from build123d import *

# Parameters (mm, degrees)
SKETCH1_R           = 35.00000000000001
BOSS_EXTRUDE1_DEPTH = 12
SKETCH2_R           = 38
CUT_EXTRUDE1_DEPTH  = 7.825
SKETCH3_R           = 40.5
CUT_EXTRUDE2_DEPTH  = 5
BOSS_EXTRUDE3_START = -3
SKETCH4_R           = 50.000000000000014
SKETCH4_R_2         = 40.5
BOSS_EXTRUDE3_DEPTH = 3
FILLET1_R           = 10
SKETCH5_R           = 2.5000000000000018
CUT_EXTRUDE3_DEPTH  = 72.72168430816446
CUT_EXTRUDE4_REACH  = 73.722
SKETCH9_R           = 3.999999999999999
CHAMFER2_SIZE       = 2.5
CHAMFER2_SIZE2      = 5.361267301273932
SKETCH10_R          = 2.499999999999999
SKETCH10_R_2        = 2.5000000000000004
SKETCH10_R_3        = 2.5000000000000018
SKETCH10_R_4        = 2.499999999999998
CUT_EXTRUDE5_DEPTH  = 7


with BuildPart() as part:
    # Sketch1 → Boss-Extrude1 (new body)
    with BuildSketch(Plane(origin=(0, 0, 0), x_dir=(0, 0, -1), z_dir=(1, 0, 0))):
        with BuildLine():
            Line((-0.9297857327654514, 49.99135423741935), (0.9297857327657116, 49.99135423741935))
            ThreePointArc((0.9297857327657116, 49.99135423741935), (50, 4.17e-15), (0.9297857327657116, -49.99135423741935))
            Line((0.9297857327657116, -49.99135423741935), (-0.9297857327654514, -49.99135423741935))
            ThreePointArc((-0.9297857327654514, -49.99135423741935), (-50.00000000000001, 1.029e-14), (-0.9297857327654514, 49.99135423741935))
        make_face()
        Circle(SKETCH1_R, mode=Mode.SUBTRACT)
    extrude(amount=BOSS_EXTRUDE1_DEPTH)

    # Sketch2 → Cut-Extrude1 (cut)
    with BuildSketch(Plane(origin=(12, 0, 0), x_dir=(0, 0, -1), z_dir=(1, 0, 0))):
        Circle(SKETCH2_R)
    extrude(amount=-CUT_EXTRUDE1_DEPTH, mode=Mode.SUBTRACT)

    # Sketch3 → Cut-Extrude2 (cut)
    with BuildSketch(Plane(origin=(12, 0, 0), x_dir=(0, 0, -1), z_dir=(1, 0, 0))):
        Circle(SKETCH3_R)
    extrude(amount=-CUT_EXTRUDE2_DEPTH, mode=Mode.SUBTRACT)

    # Sketch4 → Boss-Extrude3 (add)
    with BuildSketch(Plane(origin=(12, 0, 0), x_dir=(0, 0, -1), z_dir=(1, 0, 0)).offset(BOSS_EXTRUDE3_START)):
        with Locations(Location((0, 0, 0), (0, 0, 91.065517382))):
            Circle(SKETCH4_R)
        Circle(SKETCH4_R_2, mode=Mode.SUBTRACT)
    extrude(amount=BOSS_EXTRUDE3_DEPTH)

    # Fillet1
    # the kernel refuses this fillet: 10 mm, written as the material it takes off along each edge
    with BuildSketch(Plane(origin=(-0.2743909200605188, 49.99135423741935, 0.9297857327658466), x_dir=(0, 0, -1), z_dir=(1, 0, 0))) as fillet1_piece_1:
        with BuildLine():
            CenterArc((0.09816907994918522, -10), FILLET1_R, 90, 1.1912889407278016)
            ThreePointArc((-0.10973508325497316, -0.00216144064516044), (-0.05486813470735008, -0.0010506100030554), (0, 0))
            Line((0, 0), (0.09816907994918522, 0))
        make_face()
    extrude(amount=9.27439092006841, mode=Mode.SUBTRACT)
    with BuildSketch(Plane(origin=(-0.27439092006290455, 49.99135423741935, -0.9297857327660938), x_dir=(0, 0, 1), z_dir=(1, 0, 0))) as fillet1_piece_2:
        with BuildLine():
            CenterArc((0.09816907994990931, 10), FILLET1_R, 268.80871105927287, 1.1912889407271336)
            ThreePointArc((-0.10973508325413761, 0.00216144064516044), (-0.05486813470693486, 0.0010506100030554), (0, 0))
            Line((0, 0), (0.09816907994990931, 0))
        make_face()
    extrude(amount=9.274390920070795, mode=Mode.SUBTRACT)
    with BuildSketch(Plane(origin=(-0.27439092006166854, -49.991354237419344, -0.9297857327653347), x_dir=(0, 0.019693077349376736, -0.9998060725483275), z_dir=(1, 0, 0))) as fillet1_piece_3:
        with BuildLine():
            CenterArc((0.09878073122404785, 9.999993976768026), FILLET1_R, 268.8715968385298, 1.19128894072702)
            Line((-0.09815004226971198, 0.00193325128475002), (0, 0))
            ThreePointArc((0, 0), (0.05487818401377818, -3.011615987851e-05), (0.10975636802755673, 0))
        make_face()
    extrude(amount=9.274390920069559, mode=Mode.SUBTRACT)
    with BuildSketch(Plane(origin=(-0.27439092005998433, -49.991354237419344, 0.9297857327658335), x_dir=(0, 0.019693077349452987, 0.999806072548326), z_dir=(1, 0, 0))) as fillet1_piece_4:
        with BuildLine():
            CenterArc((0.09878073122379578, -9.999993976768023), FILLET1_R, 89.93711422074833, 1.191288940726281)
            Line((-0.09815004227073397, -0.00193325128476343), (0, 0))
            ThreePointArc((0, 0), (0.05487818401320508, 3.011615987141e-05), (0.10975636802641013, 0))
        make_face()
    extrude(amount=9.274390920067875, mode=Mode.SUBTRACT)

    # Sketch5 → Cut-Extrude3 (cut, through all)
    with BuildSketch(Plane(origin=(12, 0, 0), x_dir=(0, 0, -1), z_dir=(1, 0, 0))):
        with Locations((39.999999999999986, 9.000000000000002)):
            Circle(SKETCH5_R)
        with Locations((39.999999999999986, -8.999999999999998)):
            Circle(SKETCH5_R)
        with Locations((-40.000000000000014, -8.999999999999998)):
            Circle(SKETCH5_R)
        with Locations((-40.000000000000014, 8.999999999999998)):
            Circle(SKETCH5_R)
    extrude(amount=-CUT_EXTRUDE3_DEPTH, mode=Mode.SUBTRACT)

    # Cut-Extrude4: up to this face of the body (flat: up to its plane)
    cut_extrude4_end = Plane(part.part.faces().sort_by_distance((4.175, 0, 36.925197693))[0])
    # Sketch9 → Cut-Extrude4 (cut, up to the picked face)
    with BuildSketch(Plane(origin=(12, 0, 0), x_dir=(0, 0, -1), z_dir=(1, 0, 0)), mode=Mode.PRIVATE) as cut_extrude4_sk1:
        with Locations((-40.000000000000014, 8.999999999999998)):
            Circle(SKETCH9_R)
    cut_extrude4_tool1 = split(extrude(cut_extrude4_sk1.sketch, amount=-CUT_EXTRUDE4_REACH, mode=Mode.PRIVATE), bisect_by=cut_extrude4_end, keep=Keep.BOTH, mode=Mode.PRIVATE)
    # Sketch9 → Cut-Extrude4 (cut, up to the picked face)
    with BuildSketch(Plane(origin=(12, 0, 0), x_dir=(0, 0, -1), z_dir=(1, 0, 0)), mode=Mode.PRIVATE) as cut_extrude4_sk2:
        with Locations((-40.000000000000014, -8.999999999999998)):
            Circle(SKETCH9_R)
    cut_extrude4_tool2 = split(extrude(cut_extrude4_sk2.sketch, amount=-CUT_EXTRUDE4_REACH, mode=Mode.PRIVATE), bisect_by=cut_extrude4_end, keep=Keep.BOTH, mode=Mode.PRIVATE)
    # Sketch9 → Cut-Extrude4 (cut, up to the picked face)
    with BuildSketch(Plane(origin=(12, 0, 0), x_dir=(0, 0, -1), z_dir=(1, 0, 0)), mode=Mode.PRIVATE) as cut_extrude4_sk3:
        with Locations((39.999999999999986, -8.999999999999998)):
            Circle(SKETCH9_R)
    cut_extrude4_tool3 = split(extrude(cut_extrude4_sk3.sketch, amount=-CUT_EXTRUDE4_REACH, mode=Mode.PRIVATE), bisect_by=cut_extrude4_end, keep=Keep.BOTH, mode=Mode.PRIVATE)
    # Sketch9 → Cut-Extrude4 (cut, up to the picked face)
    with BuildSketch(Plane(origin=(12, 0, 0), x_dir=(0, 0, -1), z_dir=(1, 0, 0)), mode=Mode.PRIVATE) as cut_extrude4_sk4:
        with Locations((39.999999999999986, 8.999999999999998)):
            Circle(SKETCH9_R)
    cut_extrude4_tool4 = split(extrude(cut_extrude4_sk4.sketch, amount=-CUT_EXTRUDE4_REACH, mode=Mode.PRIVATE), bisect_by=cut_extrude4_end, keep=Keep.BOTH, mode=Mode.PRIVATE)
    add(cut_extrude4_tool1.solids().sort_by(Axis((12, 9, 40), (-1, 0, 0)))[0], mode=Mode.SUBTRACT)
    add(cut_extrude4_tool2.solids().sort_by(Axis((12, -9, 40), (-1, 0, 0)))[0], mode=Mode.SUBTRACT)
    add(cut_extrude4_tool3.solids().sort_by(Axis((12, -9, -40), (-1, 0, 0)))[0], mode=Mode.SUBTRACT)
    add(cut_extrude4_tool4.solids().sort_by(Axis((12, 9, -40), (-1, 0, 0)))[0], mode=Mode.SUBTRACT)

    # Chamfer2
    chamfer2_edges = [part.edges().sort_by_distance(p)[0] for p in [
        (0, 4.163e-14, 50.000000000000014),
        (0, 8.2534e-13, -50),
        (0, 49.99135423741935, 4.9938e-13),
        (0, -49.99135423741935, 7.583e-14),
        (0, -49.99081386265752, 0.9355743520296814),
        (0, -49.990813862657504, -0.9355743520294721),
        (0, 49.99081386265747, -0.9355743520297026),
        (0, 49.99081386265747, 0.9355743520307873),
    ]]
    chamfer2_side = [part.faces().sort_by_distance(p)[0] for p in [
        (0, -48.576798978470165, -0.920873784247004),
    ]]
    chamfer(chamfer2_edges, length=CHAMFER2_SIZE, length2=CHAMFER2_SIZE2, reference=chamfer2_side[0])

    # Sketch10 → Cut-Extrude5 (cut)
    with BuildSketch(Plane(origin=(12, 0, 0), x_dir=(0, 0, -1), z_dir=(1, 0, 0))):
        with Locations((-31.819805153394583, 31.819805153394686)):
            Circle(SKETCH10_R)
        with Locations((31.819805153394796, 31.81980515339447)):
            Circle(SKETCH10_R_2)
        with Locations((31.81980515339436, -31.819805153394906)):
            Circle(SKETCH10_R_3)
        with Locations((-31.81980515339502, -31.81980515339425)):
            Circle(SKETCH10_R_4)
    extrude(amount=-CUT_EXTRUDE5_DEPTH, mode=Mode.SUBTRACT)


solid = part.part
Build history of the part. All positions in model axes, mm. A direction names the side the tool comes from. Coordinates: 2 decimals unless noted, no trailing zeros. One line per item, written item: value.
(1) Mould opens along Z. For faces 1 (the flat face through (2.72, 48.76, 0.01)), 2 (the flat face through (7, -39, 0)) say: pulls with the +Z half, pulls with the -Z half, needs draft (parallel to the pull), parting line crosses it, or undercut.
Checked values:
face 1: needs draft
face 2: undercut
(2) Tool access for faces 3 (the flat face through (5, -32, -32)), 4 (the flat face through (2.72, -48.76, -0.01)): list every direction of +Z, -Z, +X, -X, +Y, -Y with a clear straight run to the whole face (end or side of a thin tool).
Checked values:
face 3: +X
face 4: +Z, -Z, -X, -Y
(3) Drop flat-ended pins along their axis: pin 1 Ø4 at (y, z) = (-8, 39.5) entering from +X (3 decimals); pin 2 Ø4 at (x, y) = (3, 16.5) entering from +Z; pin 3 Ø1.5 at (y, z) = (1, 39) entering from +X. Give the stop position or say it passes through.
Checked values:
pin 1: x = 4.175
pin 2: z = 47.23
pin 3: x = 7
(4) Probe line 1 (Y direction, x = 6.25, z = 43.5); line 2 (Z direction, x = 8.5, y = 1); line 3 (Z direction, x = 5.5, y = -5.5). List the from-to ranges inside material, lowest first. Write a range as [from, to].
Checked values:
line 1: [-24.65, -10.94], [-7.06, 7.06], [10.94, 24.65]
line 2: [-49.99, -40.49], [40.49, 49.99]
line 3: [-49.7, -41.94], [-38.06, -37.6], [37.6, 38.06], [41.94, 49.7]
